For this review, take the finished solid that the model builds, in its own axes (mm). A direction names the side the tool comes from. Coordinates: 2 decimals unless noted, no trailing zeros. Loops run counter-clockwise (first coordinate to the right, second up) from the corner with the lowest first, then second, coordinate; pieces in that order, holes last. Notation, with made-up numbers: M 62.5,-16 L 68.5,-16 A17 ccw 68.5,4 Z; hole C -37.5,-37 d1. An arc over 180 degrees is marked long. Write item = value, one per line.
from build123d import *

# Parameters (mm, degrees)
SKETCH_W        = 117
SKETCH_H        = 35
PAD_DEPTH       = 35
SKETCH001_R     = 15
POCKET_DEPTH    = 97
SKETCH002_R     = 7.5
POCKET001_DEPTH = 12.5
SKETCH003_R     = 6
POCKET002_DEPTH = 12.5
SKETCH004_R     = 1.25
HOLE_DEPTH      = 117.001
SKETCH005_R     = 1.25
HOLE001_DEPTH   = 25
HOLE001_TIPS_R  = 1.25
SKETCH006_R     = 1.5
HOLE002_DEPTH   = 25
HOLE002_TIPS_R  = 1.5


with BuildPart() as part:
    # Sketch → Pad (new body)
    with BuildSketch(Plane.XZ):
        with Locations((58.5, 17.5)):
            Rectangle(SKETCH_W, SKETCH_H)
    extrude(amount=PAD_DEPTH)

    # Sketch001 → Pocket (cut)
    with BuildSketch(Plane(origin=(0, 0, 0), x_dir=(0, 0, -1), z_dir=(-1, 0, 0))):
        with Locations((-17.5, 17.5)):
            Circle(SKETCH001_R)
    extrude(amount=-POCKET_DEPTH, mode=Mode.SUBTRACT)

    # Sketch002 → Pocket001 (cut)
    with BuildSketch(Plane(origin=(120, 0, 0), x_dir=(0, 0, 1), z_dir=(1, 0, 0))):
        with Locations((17.25, 17.25)):
            Circle(SKETCH002_R)
    extrude(amount=-POCKET001_DEPTH, mode=Mode.SUBTRACT)

    # Sketch003 → Pocket002 (cut)
    with BuildSketch(Plane(origin=(97, 0, 0), x_dir=(0, 0, -1), z_dir=(-1, 0, 0))):
        with Locations((-17.5, 17.5)):
            Circle(SKETCH003_R)
    extrude(amount=-POCKET002_DEPTH, mode=Mode.SUBTRACT)

    # Sketch004 → Hole (cut, through all)
    with BuildSketch(Plane(origin=(0, 0, 0), x_dir=(0, 0, -1), z_dir=(-1, 0, 0))):
        with Locations((-31, 4)):
            Circle(SKETCH004_R)
        with Locations((-4, 31)):
            Circle(SKETCH004_R)
    extrude(amount=-HOLE_DEPTH, mode=Mode.SUBTRACT)

    # Sketch005 (on Face2 of Hole) → Hole001 (cut)
    with BuildSketch(Plane(origin=(0, 0, 0), x_dir=(0, 0, -1), z_dir=(-1, 0, 0))):
        with Locations((-4, 4)):
            Circle(SKETCH005_R)
        with Locations((-31, 31)):
            Circle(SKETCH005_R)
    extrude(amount=-HOLE001_DEPTH, mode=Mode.SUBTRACT)

    # Hole001 tips → Hole001 tip 1 section 0
    with BuildSketch(Plane(origin=(25, 0, 0), x_dir=(0, 0, -1), z_dir=(-1, 0, 0)), mode=Mode.PRIVATE) as hole001_tip_1_s0:
        with Locations((-4, 4)):
            Circle(HOLE001_TIPS_R)
    loft([hole001_tip_1_s0.sketch, Vertex(25.751076, -4, 4)], mode=Mode.SUBTRACT)

    # Hole001 tips → Hole001 tip 2 section 0
    with BuildSketch(Plane(origin=(25, 0, 0), x_dir=(0, 0, -1), z_dir=(-1, 0, 0)), mode=Mode.PRIVATE) as hole001_tip_2_s0:
        with Locations((-31, 31)):
            Circle(HOLE001_TIPS_R)
    loft([hole001_tip_2_s0.sketch, Vertex(25.751076, -31, 31)], mode=Mode.SUBTRACT)

    # Sketch006 → Hole002 (cut)
    with BuildSketch(Plane(origin=(117, 0, 0), x_dir=(0, 0, 1), z_dir=(1, 0, 0))):
        with Locations((31, 17.5)):
            Circle(SKETCH006_R)
    extrude(amount=-HOLE002_DEPTH, mode=Mode.SUBTRACT)

    # Hole002 tips → Hole002 tip 1 section 0
    with BuildSketch(Plane(origin=(92, 0, 0), x_dir=(0, 0, 1), z_dir=(1, 0, 0)), mode=Mode.PRIVATE) as hole002_tip_1_s0:
        with Locations((31, 17.5)):
            Circle(HOLE002_TIPS_R)
    loft([hole002_tip_1_s0.sketch, Vertex(91.098709, -17.5, 31)], mode=Mode.SUBTRACT)


solid = part.part
Q1. Add section B-B (z = 26.5). Write out the cut boundary in (x, y).
Solved:
outline = M 0,-35 L 117,-35 L 117,0 L 0,0 L 0,-5.5 L 97,-5.5 L 97,-29.5 L 0,-29.5 Z
Q2. Draft analysis for pull direction Z (two halves, no side actions). For faces 1 (the face through (12.32, -2.78, 4.27)), 2 (the face through (58, -17, 35)), 3 (the face through (25.631, -3.924, 3.816)), 4 (the face through (0, -33, 17)), state which applies: +Z half, -Z half, draft (parallel to the pull), parting line (faces both ways), or undercut.
Solved:
face_1 = undercut
face_2 = +Z half
face_3 = undercut
face_4 = draft
Q3. For pin 1 Ø4.5 at (y, z) = (-21, 15) entering from +X; pin 2 Ø1.5 at (y, z) = (-25, 26.5) entering from -X, all flat-tipped, find the tip position at first contact; note any pin that passes through.
Solved:
pin_1 = 107.5
pin_2 = 97
Q4. For line 1 along Y through (x, z) = (70, 17); line 2 along Z through (x, y) = (7.5, -4.5); line 3 along Z through (x, y) = (6, -17), list the stretches that pass through material, from the lowest coordinate up.
Solved:
line_1 = -35 to -32.49, -2.51 to 0
line_2 = 0 to 2.85, 5.15 to 10.02, 24.98 to 29.85, 32.15 to 35
line_3 = 0 to 2.51, 32.49 to 35
Q5. Add section C-C (y = -26). Write out the cut boundary in (x, z), and give its area (3 significant figures).
Solved:
outline = M 0,0 L 117,0 L 117,35 L 0,35 L 0,29.86 L 97,29.86 L 97,5.14 L 0,5.14 Z
area = 1,700 mm²
Q6. Machinability: for faces 5 (the face through (58, -35, 18)), 6 (the face through (12.325, -30.521, 29.845)), 7 (the face through (112.316, -22.319, 11.722)), which of the approach directions +Z, -Z, +X, -X, +Y, -Y give a long, thin tool a straight path to every point of the face, cutting with its end or side? Answer none if there is none.
Solved:
face_5 = +Z, -Z, +X, -X, -Y
face_6 = -X
face_7 = +X
Q7. Add section A-A (z = 17.5). Write out the cut boundary in (x, y), and give its area (3 significant figures).
Solved:
outline = M 0,-35 L 117,-35 L 117,-24.75 L 107.5,-24.75 L 107.5,-23.5 L 97,-23.5 L 97,-32.5 L 0,-32.5 Z; M 0,-2.5 L 97,-2.5 L 97,-11.5 L 107.5,-11.5 L 107.5,-9.75 L 117,-9.75 L 117,0 L 0,0 Z
area = 917 mm²
